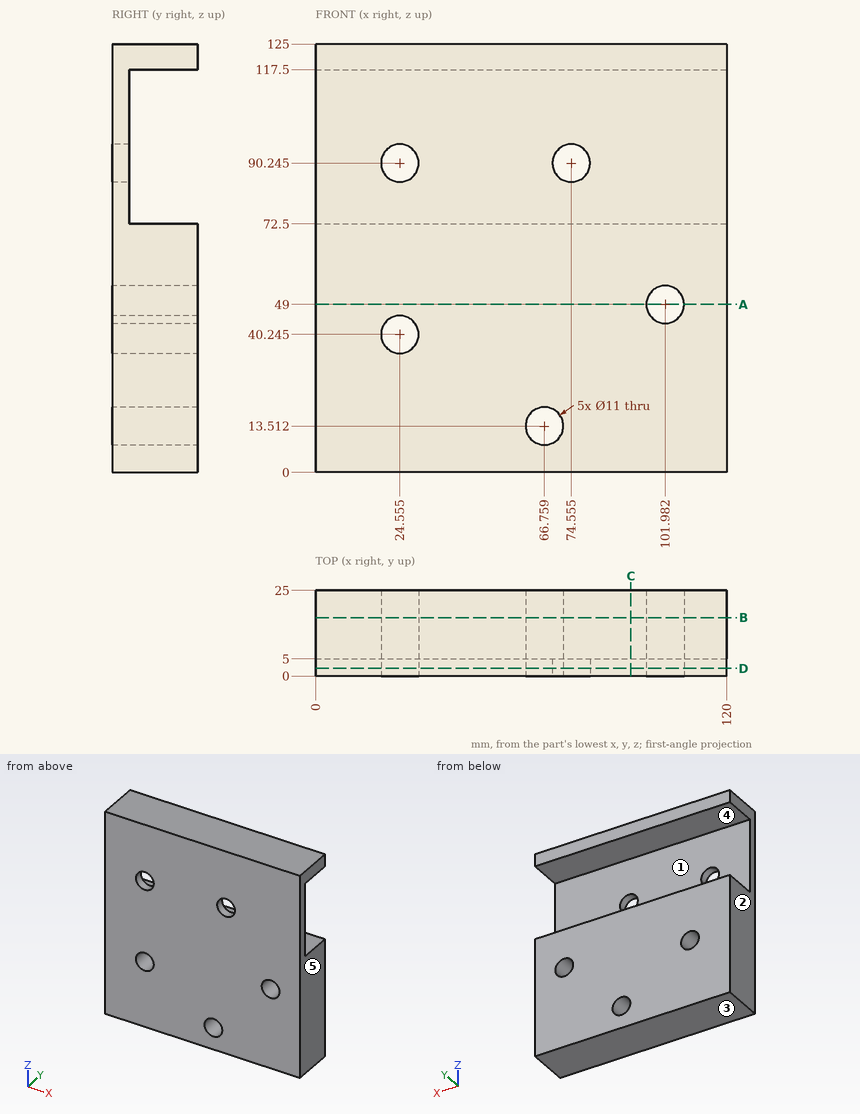
Could you check a few things on this drawing? It's one solid part, dimensions in mm from its lowest x, y, z. A direction names the side the tool comes from. Round coordinates to 2 decimals unless told otherwise and drop trailing zeros. Order: outer loops, then holes, each group sorted by start corner. A loop starts at its lowest first (then second) coordinate and runs counter-clockwise, first axis right, second up. Notation, with made-up numbers: M 37.25,0 L 81.25,0 A20 cw 81.25,8 Z; hole C 86.25,65 d6. An arc over 180 degrees is marked long. One line per question, with ' | ' between items. Start each with the question number.
(1) Suppose I cut it at C-C on x = 92. List the corners of the cut face in (y, z) for me.
(2) Please list where these lines run through material, in increasing order: line 1 along Z through (x, y) = (32, 16); line 2 along Z through (x, y) = (71.5, 24) (1 decimal); line 3 along Z through (x, y) = (71, 8.25) (1 decimal).
(3) Suppose I cut it at D-D on y = 2.25. List the corners of the cut face in (x, z) for me (1 decimal).
(4) Thinking about a two-plate mould opening in Z: for the marked faces 3, 4 and 5, which applies, +Z half, -Z half, draft (parallel to the pull), parting line (faces both ways), or undercut?
(5) Suppose I cut it at B-B on y = 17. List the corners of the cut face in (x, z) for me (1 decimal).
(6) Suppose I cut it at A-A on z = 49. List the corners of the cut face in (x, y) for me.
(7) For P1, Ø5, axis at x = 105.5, y = 4, coming from the -Z side, with a flat end and sliding along its axis, tell me the tip position at first contact or that it passes through.
(8) For the marked faces 1 and 2, which set-ups out of +Z, -Z, +X, -X, +Y, -Y let a thin tool reach every point of the face, with its end or its side?
Geometry results:
1) outline: M 0,0 L 25,0 L 25,72.5 L 5,72.5 L 5,117.5 L 25,117.5 L 25,125 L 0,125 Z
2) line 1: 0 to 72.5, 117.5 to 125 | line 2: 0 to 10.7, 16.3 to 72.5, 117.5 to 125 | line 3: 0 to 10, 17 to 72.5, 117.5 to 125
3) outline: M 0,0 L 120,0 L 120,125 L 0,125 Z; hole C 24.6,40.2 d11; hole C 24.6,90.2 d11; hole C 66.8,13.5 d11; hole C 74.6,90.2 d11; hole C 102,49 d11
4) face 3: -Z half | face 4: undercut | face 5: draft
5) outline: M 0,0 L 120,0 L 120,72.5 L 0,72.5 Z; M 0,117.5 L 120,117.5 L 120,125 L 0,125 Z; hole C 24.6,40.2 d11; hole C 66.8,13.5 d11; hole C 102,49 d11
6) outline: M 0,0 L 96.48,0 L 96.48,25 L 0,25 Z; M 107.48,0 L 120,0 L 120,25 L 107.48,25 Z
7) P1: z = 0
8) face 1: +X, -X, +Y | face 2: +Z, -Z, -X, +Y, -Y
